Drawing for the job (mm, zero at the part's lowest x, y, z). A direction names the side the tool comes from. Round coordinates to 2 decimals unless told otherwise and drop trailing zeros. Order: outer loops, then holes, each group sorted by start corner. A loop starts at its lowest first (then second) coordinate and runs counter-clockwise, first axis right, second up. Notation, with made-up numbers: (-19, -30) - (1, -30) arc R25 cw to (1, 7) - close; hole circle Ø2 at (53, 19). An arc over 180 degrees is marked (long way). Put each result on its own line as item: value. Start each with the question number.
Item 1: Mould opens along Z. For the marked faces 1, 2 and 3 say: pulls with the +Z half, pulls with the -Z half, needs draft (parallel to the pull), parting line crosses it, or undercut.
Item 2: Saw through at A-A on z = 7.5. List the corners of the cut face in (x, y), plus the area to 3 significant figures.
Item 3: Saw through at C-C on x = 7.5. List the corners of the cut face in (y, z), plus the area to 3 significant figures.
Item 4: Saw through at B-B on y = 1.5. List the corners of the cut face in (x, z).
Item 5: Probe probe 1 along Z at (x, y) = (7.5, 8.75); probe 2 along Y at (x, z) = (4, 4.5); probe 3 along Z at (x, y) = (9.5, 2.5). List the from-to ranges inside material, lowest first.
Item 6: Saw through at D-D on y = 8.5. List the corners of the cut face in (x, z).
Item 7: Which spindle directions (+Z, -Z, +X, -X, +Y, -Y) get a long thin tool onto all of the face, cutting with end or side? Do the marked faces 4, 5 and 6. Say none if no direction does.
Item 8: Pin check, flat tips, straight feed: pin 1 Ø5 at (x, y) = (10, 8.5) entering from +Z; pin 2 Ø0.6 at (x, z) = (4, 8) entering from -Y; pin 3 Ø4 at (x, y) = (13, 8) entering from -Z; pin 4 Ø0.6 at (x, y) = (9, 1) entering from +Z. Stop position of each tip, or through.
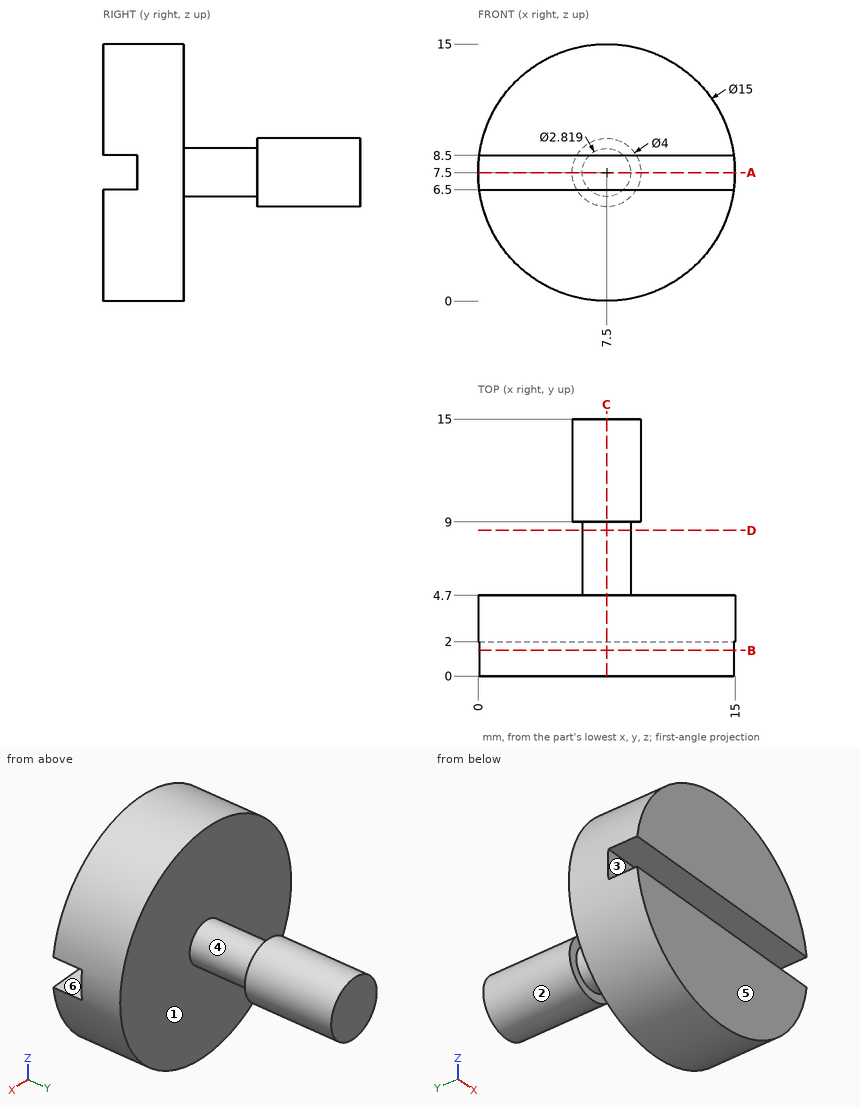
Results found:
1. face 1: needs draft
1. face 2: parting line crosses it
1. face 3: undercut
2. outline: (0, 2) - (15, 2) - (15, 4.7) - (8.91, 4.7) - (8.91, 9) - (9.5, 9) - (9.5, 15) - (5.5, 15) - (5.5, 9) - (6.09, 9) - (6.09, 4.7) - (0, 4.7) - close
2. area: 76.6 mm²
3. outline: (0, 0) - (4.7, 0) - (4.7, 6.09) - (9, 6.09) - (9, 5.5) - (15, 5.5) - (15, 9.5) - (9, 9.5) - (9, 8.91) - (4.7, 8.91) - (4.7, 15) - (0, 15) - (0, 8.5) - (2, 8.5) - (2, 6.5) - (0, 6.5) - close
3. area: 103 mm²
4. outline: (0.07, 6.5) arc R7.5 ccw to (14.93, 6.5) - close; (0.07, 8.5) - (14.93, 8.5) arc R7.5 ccw to start
5. probe 1: z = 6.09 to 8.91
5. probe 2: y = 0 to 4.7
5. probe 3: z = 0.27 to 14.73
6. outline: circle Ø2.82 at (7.5, 7.5)
7. face 4: none
7. face 5: +Z, -Z, +X, -X, -Y
7. face 6: +X, -X, -Y
8. pin 1: stops at z = 9.5
8. pin 2: stops at y = 2
8. pin 3: passes through
8. pin 4: stops at z = 14.9
